```python
from build123d import *

# Parameters (mm, degrees)
SKETCH1_W             = 110
SKETCH1_H             = 70
PLATE_DEPTH           = 4
SKETCH2_W             = 97.2
SKETCH2_H             = 40
SCREEN_HOLE_DEPTH     = 66.314623171
F_3_0MM_DOWEL_HOLE1_D = 3
SKETCH6_W             = 80
SKETCH6_H             = 15
CUT_EXTRUDE1_DEPTH    = 66.314623171


with BuildPart() as part:
    # Sketch1 → Plate (new body)
    with BuildSketch(Plane.XY):
        Rectangle(SKETCH1_W, SKETCH1_H)
    extrude(amount=PLATE_DEPTH)

    # Sketch2 → Screen hole (cut, through all)
    with BuildSketch(Plane(origin=(0, 0, 0), x_dir=(-1, 0, 0), z_dir=(0, 0, -1))):
        Rectangle(SKETCH2_W, SKETCH2_H)
    extrude(amount=-SCREEN_HOLE_DEPTH, mode=Mode.SUBTRACT)

    # Ø3.0mm Dowel Hole1 (through all)
    with Locations(Plane(origin=(46.5, 27.5, 0), x_dir=(-1, 0, 0), z_dir=(0, 0, -1))):
        with Locations((0, 0), (93, 0), (93, -55), (0, -55)):
            Hole(F_3_0MM_DOWEL_HOLE1_D / 2)

    # Sketch6 → Cut-Extrude1 (cut, through all)
    with BuildSketch(Plane(origin=(0, 0, 0), x_dir=(-1, 0, 0), z_dir=(0, 0, -1))):
        with Locations((0, 27.5)):
            Rectangle(SKETCH6_W, SKETCH6_H)
    extrude(amount=-CUT_EXTRUDE1_DEPTH, mode=Mode.SUBTRACT)


solid = part.part
```
Model file for the job. Use its own axes, mm. A direction names the side the tool comes from. Give positions to 0.01 mm unless a question says otherwise; leave off trailing zeros. Loops run counter-clockwise (first coordinate to the right, second up) from the corner with the lowest first, then second, coordinate; pieces in that order, holes last. Notation, with made-up numbers: M 33,4 L 87,4 A14 ccw 87,20 Z; hole C -23,-29 d6. An arc over 180 degrees is marked long. Use one line per item in the form item = value.
Item 1: Two-plate mould, pull along Y, no slides. Class faces 4 (the flat face through (-1, -35, 2)), 5 (the flat face through (-44, 20, 2)), 6 (the flat face through (47, 35, 2)), 7 (the flat face through (0, -23, 0)): released by +Y, released by -Y, zero draft, split by the parting line, or undercut.
Filled in:
face_4 = released by -Y
face_5 = undercut
face_6 = released by +Y
face_7 = zero draft
Item 2: Slice it at C-C on z = 3.05. List the corners of the cut face in (x, y).
Filled in:
outline = M -55,-35 L 55,-35 L 55,35 L 40,35 L 40,20 L 48.6,20 L 48.6,-20 L -48.6,-20 L -48.6,20 L -40,20 L -40,35 L -55,35 Z; hole C -46.5,-27.5 d3; hole C -46.5,27.5 d3; hole C 46.5,-27.5 d3; hole C 46.5,27.5 d3
Item 3: Slice it at B-B on x = -46.5. List the corners of the cut face in (y, z), and give its area (3 significant figures).
Filled in:
outline = M -35,0 L -29,0 L -29,4 L -35,4 Z; M -26,0 L -20,0 L -20,4 L -26,4 Z; M 20,0 L 26,0 L 26,4 L 20,4 Z; M 29,0 L 35,0 L 35,4 L 29,4 Z
area = 96.0 mm^2
Item 4: Slice it at A-A on y = -27.5. List the corners of the cut face in (x, z).
Filled in:
outline = M -55,0 L -48,0 L -48,4 L -55,4 Z; M -45,0 L 45,0 L 45,4 L -45,4 Z; M 48,0 L 55,0 L 55,4 L 48,4 Z
Item 5: Which spindle directions (+Z, -Z, +X, -X, +Y, -Y) get a long thin tool onto all of the face, cutting with end or side? Do faces 1 (the flat face through (-40, 27, 2)), 2 (the flat face through (44, 20, 2)), 3 (the flat face through (0, -23, 4)). Say none if no direction does.
Filled in:
face_1 = +Z, -Z, +Y
face_2 = +Z, -Z
face_3 = +Z, +X, -X, +Y, -Y
Item 6: Drill centre lines: L1, parallel to Y at x = 46.5, z = 0.95; L2, parallel to X at y = 2, z = 3.5; L3, parallel to X at y = 26.5, z = 2.2. Where is each one in solid material? Low to high.
Filled in:
L1 = -35 to -29, -26 to -20, 20 to 26, 29 to 35
L2 = -55 to -48.6, 48.6 to 55
L3 = -55 to -47.62, -45.38 to -40, 40 to 45.38, 47.62 to 55
Item 7: Slice it at D-D on y = -4. List the corners of the cut face in (x, z).
Filled in:
outline = M -55,0 L -48.6,0 L -48.6,4 L -55,4 Z; M 48.6,0 L 55,0 L 55,4 L 48.6,4 Z
